Here's the drawing with two shaded views (mm, measured from the low corner). I have some questions. Give positions to 0.01 mm unless a question says otherwise; leave off trailing zeros. Write each loop counter-clockwise with the first axis right and the second up, starting at its lowest first coordinate (ties: lowest second). Pieces come first, ordered by that corner, then holes. Notation, with made-up numbers: (44.5, 11.25) - (54.5, 11.25) arc R29 cw to (54.5, 41.25) - close; hole circle Ø2 at (47.5, -1). An arc over 180 degrees is marked (long way). Use one line per item in the form item = value.
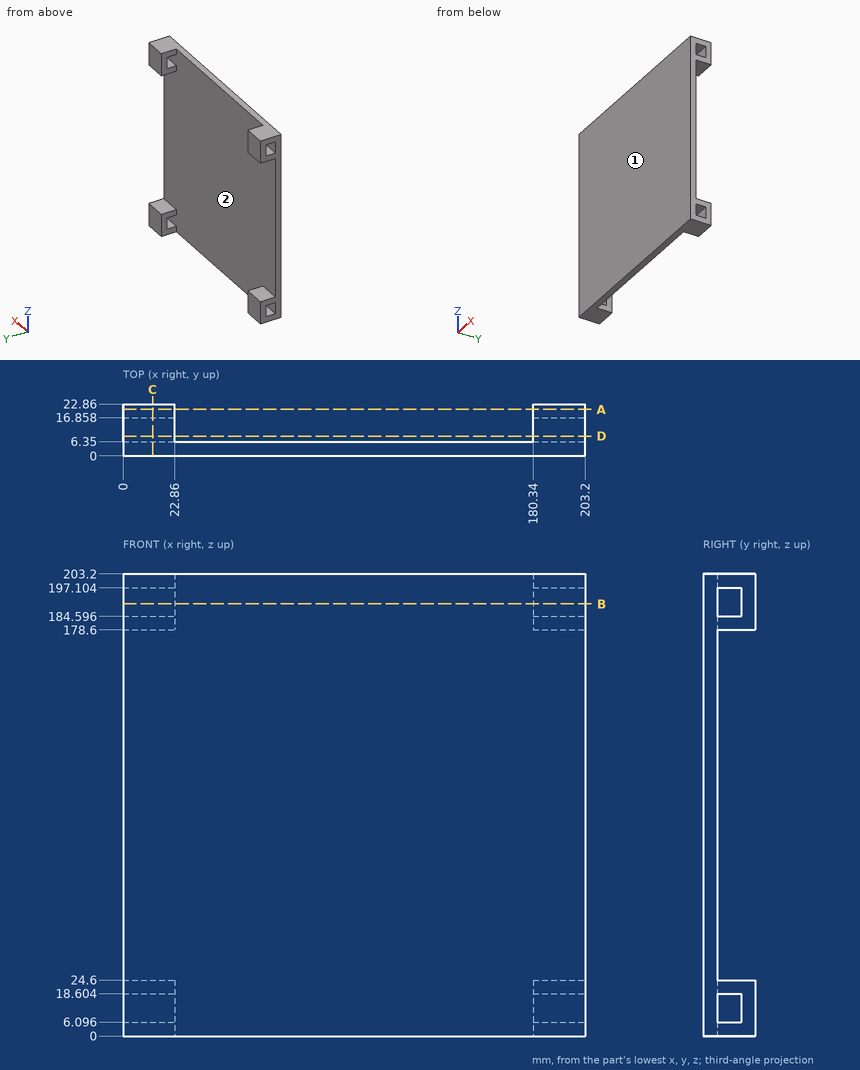
1. Imagine slicing it at A-A, the plane y = 20.5. List the corners of the cut face in (x, z) for me, and give its area (3 significant figures).
Response values:
outline = (0, 0) - (22.86, 0) - (22.86, 24.6) - (0, 24.6) - close; (0, 178.6) - (22.86, 178.6) - (22.86, 203.2) - (0, 203.2) - close; (180.34, 0) - (203.2, 0) - (203.2, 24.6) - (180.34, 24.6) - close; (180.34, 178.6) - (203.2, 178.6) - (203.2, 203.2) - (180.34, 203.2) - close
area = 2,250 mm²
2. Imagine slicing it at D-D, the plane y = 8.75. State how many separate pieces and enclosed holes the cut face has, and give its area (3 significant figures).
Response values:
separate_pieces = 8
enclosed_holes = 0
area = 1,110 mm²
3. Imagine slicing it at B-B, the plane z = 190. List the corners of the cut face in (x, y) for me.
Response values:
outline = (0, 0) - (203.2, 0) - (203.2, 6.35) - (0, 6.35) - close; (0, 16.86) - (22.86, 16.86) - (22.86, 22.86) - (0, 22.86) - close; (180.34, 16.86) - (203.2, 16.86) - (203.2, 22.86) - (180.34, 22.86) - close
4. Imagine slicing it at C-C, the plane x = 13. List the corners of the cut face in (y, z) for me, and give its area (3 significant figures).
Response values:
outline = (0, 0) - (22.86, 0) - (22.86, 24.6) - (6.35, 24.6) - (6.35, 178.6) - (22.86, 178.6) - (22.86, 203.2) - (0, 203.2) - close; hole (6.35, 6.1) - (16.86, 6.1) - (16.86, 18.6) - (6.35, 18.6) - close; hole (6.35, 184.6) - (16.86, 184.6) - (16.86, 197.1) - (6.35, 197.1) - close
area = 1,840 mm²
5. For pin 1 (12 mm diameter, centred on x = 148, z = 64.5, fed in from +Y), with a flat end and sliding along its axis, tell me the tip position at first contact or that it passes through.
Response values:
pin_1 = 6.35
6. If I drill on line 1 (X direction, y = 21.75, z = 15); line 2 (Y direction, x = 47, z = 115.5), over which ranges is the centre line in solid material (lowest first)? Write a range as from..to.
Response values:
line_1 = 0..22.86, 180.34..203.2
line_2 = 0..6.35
7. If we mould it in two halves opening along Z, with no side actions, what happens to the marked faces 1 and 2? For each: pulls with the +Z half, pulls with the -Z half, needs draft (parallel to the pull), parting line crosses it, or undercut.
Response values:
face_1 = needs draft
face_2 = undercut
